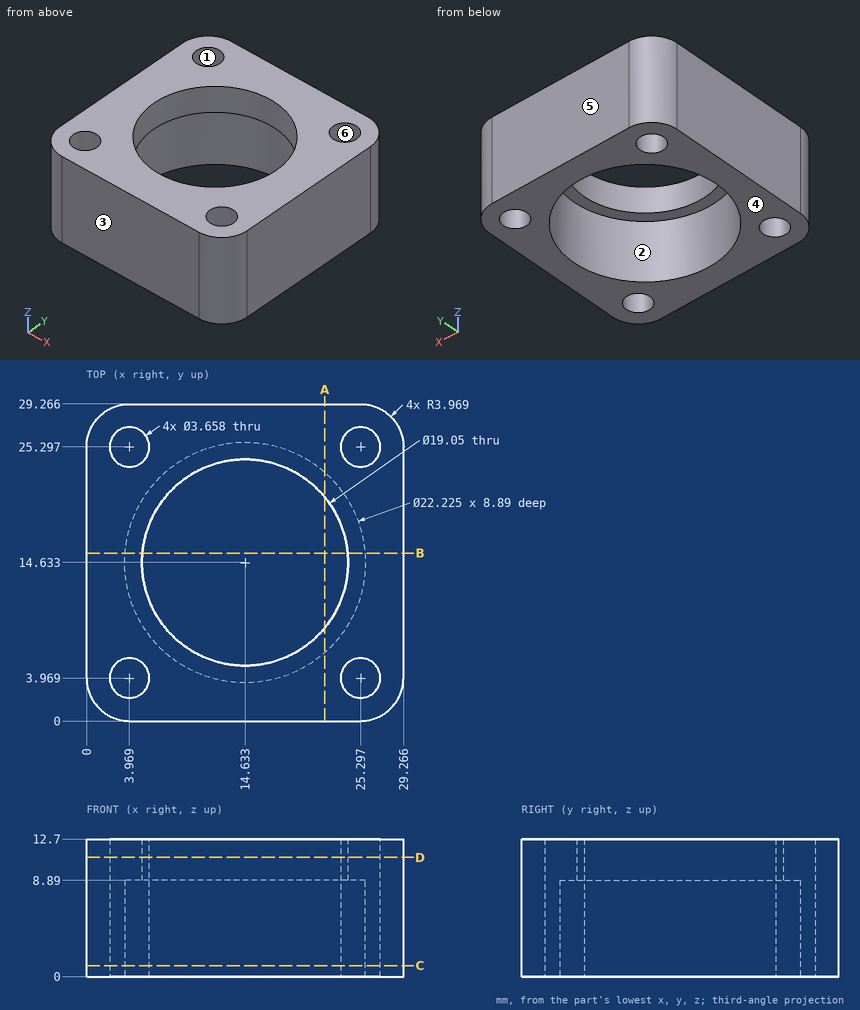
Design review of the part shown in the three views and the two pictorial views. Dimensions are in mm from the part's minimum x, y and z. A direction names the side the tool comes from. Give positions to 0.01 mm unless a question says otherwise; leave off trailing zeros. Write each loop counter-clockwise with the first axis right and the second up, starting at its lowest first coordinate (ties: lowest second). Pieces come first, ordered by that corner, then holes. Notation, with made-up numbers: M 12,66 L 68,66 A8 ccw 68,78 Z; hole C 63.25,11.5 d5. An arc over 180 degrees is marked long. Return JSON: item names as keys, results as strings. Group by question number.
Item 1: Wall thickness on line 1 along X through (y, z) = (2.5, 5.5) (1 decimal); line 2 along X through (y, z) = (15.5, 3.75) (1 decimal): over which ranges is each line inside the solid? List them lowest first.
Item 2: Tool access review of the marked faces 1 and 2: name each direction out of +Z, -Z, +X, -X, +Y, -Y from which nothing blocks a thin tool from reaching the whole face with its end or side.
Item 3: Take a section at D-D (z = 11). Count the separate pieces of the cut face and the enclosed holes in it, plus the area to 3 significant figures.
Item 4: Take a section at B-B (y = 15.5). Give the boundary of the cut face in (x, z) (1 decimal).
Item 5: Take a section at C-C (z = 1). Give the boundary of the cut face in (x, y) (1 decimal), plus the area to 3 significant figures.
Item 6: Clearance check with a flat-ended pin moving along its axis: pin 1 Ø6 at (x, y) = (20, 10) entering from -Z. State where the tip first meets the part, or that it passes through.
Item 7: Take a section at A-A (x = 22). Give the boundary of the cut face in (y, z) (1 decimal), plus the area to 3 significant figures.
Item 8: The part is to be moulded in two halves that separate along Y. For the marked faces 3, 4, 5 and 6, say which applies: pulls with the +Y half, pulls with the -Y half, needs draft (parallel to the pull), parting line crosses it, or undercut.
Return value:
{
 "1": {"line 1": "x = 0.3 to 2.9, 5.1 to 24.2, 26.4 to 29", "line 2": "x = 0 to 3.6, 25.7 to 29.3"},
 "2": {"face 1": "+Z, -Z", "face 2": "-Z"},
 "3": {"separate pieces": "1", "enclosed holes": "5", "area": "516 mm2"},
 "4": {"outline": "M 0,0 L 3.6,0 L 3.6,8.9 L 5.1,8.9 L 5.1,12.7 L 0,12.7 Z; M 24.1,8.9 L 25.7,8.9 L 25.7,0 L 29.3,0 L 29.3,12.7 L 24.1,12.7 Z"},
 "5": {"outline": "M 0,4 A4 ccw 4,0 L 25.3,0 A4 ccw 29.3,4 L 29.3,25.3 A4 ccw 25.3,29.3 L 4,29.3 A4 ccw 0,25.3 Z; hole C 4,4 d3.7; hole C 4,25.3 d3.7; hole C 14.6,14.6 d22.2; hole C 25.3,4 d3.7; hole C 25.3,25.3 d3.7", "area": "413 mm2"},
 "6": {"pin 1": "stops at z = 8.89"},
 "7": {"outline": "M 0,0 L 6.3,0 L 6.3,8.9 L 8.6,8.9 L 8.6,12.7 L 0,12.7 Z; M 20.7,8.9 L 23,8.9 L 23,0 L 29.3,0 L 29.3,12.7 L 20.7,12.7 Z", "area": "178 mm2"},
 "8": {"face 3": "pulls with the -Y half", "face 4": "needs draft", "face 5": "pulls with the +Y half", "face 6": "undercut"}
}
